from build123d import *

# Parameters (mm, degrees)
F1_DEPTH       = 31.75
F4_D           = 6.985
F4_DEPTH       = 12.7
F4_CSINK_D     = 12.7
F4_CSINK_ANGLE = 82
F4_TIP         = 2.098505712
F5_SIZE2       = 0.381
F5_SIZE        = 6.35
F2_W           = 4.7625
F2_H           = 20.32
F6_DEPTH       = 25.4
F7_SIZE2       = 5.08
F7_SIZE        = 0.381
F8_R           = 1.905
F9_T1_DEPTH    = 23.1775
F9_T3_DEPTH    = 27.94
F9_S7_W        = 1.905
F9_S7_H        = 1.905
F9_T8_DEPTH    = 1.905
F9_S13_W       = 1.905
F9_S13_H       = 1.905
F9_T14_DEPTH   = 1.905
F9_S19_W       = 1.905
F9_S19_H       = 1.905
F9_T20_DEPTH   = 1.905
F9_S25_W       = 1.905
F9_S25_H       = 1.905
F9_T26_DEPTH   = 1.905


# Not quite as in the source:
# - a fillet or chamfer that OpenCascade refuses, or shapes differently, is made with other operations: its cross-section is extruded or revolved along the edge and cut away or added


with BuildPart() as f1:
    # F0 (on Right) → F1 (new body, symmetric)
    with BuildSketch(Plane.YZ):
        Polygon((-12.7, 0), (-12.7, 20.32), (12.7, 20.32), (12.7, 0), (17.4625, 0), (17.4625, 25.0825), (-17.4625, 25.0825), (-17.4625, 0), align=None)
    extrude(amount=F1_DEPTH, both=True)

    # F4
    with Locations(Plane.XY.offset(25.0825)):
        with Locations((0, 0)):
            CounterSinkHole(F4_D / 2, F4_CSINK_D / 2, depth=F4_DEPTH, counter_sink_angle=F4_CSINK_ANGLE)
            with Locations((0, 0, -(F4_DEPTH + F4_TIP / 2))):  # 118° drill point
                Cone(0, F4_D / 2, F4_TIP, mode=Mode.SUBTRACT)

    # F5
    f5_edges = [f1.edges().sort_by_distance(p)[0] for p in [
        (0, -12.7, 0),
    ]]
    f5_side = f1.faces().sort_by_distance((0, -12.7, 10.16))[0]
    chamfer(f5_edges, length=F5_SIZE, length2=F5_SIZE2, reference=f5_side)

    # F2 (on face) → F6 (join)
    with BuildSketch(Plane(origin=(-31.75, 0, 0), x_dir=(0, -1, 0), z_dir=(-1, 0, 0))):
        with Locations((-15.08125, 10.16)):
            Rectangle(F2_W, F2_H)
    extrude(amount=F6_DEPTH)

    # F7
    f7_edges = [f1.edges().sort_by_distance(p)[0] for p in [
        (-12.7, 12.7, 0),
    ]]
    chamfer(f7_edges, length=F7_SIZE, length2=F7_SIZE2)

    # F8
    f8_edges = [f1.edges().sort_by_distance(p)[0] for p in [
        (-31.75, 0, 25.0825),
        (-31.75, 15.08125, 20.32),
        (-57.15, 15.08125, 20.32),
        (31.75, 0, 25.0825),
        (0, 17.4625, 25.0825),
        (-31.75, 17.4625, 22.70125),
        (-44.45, 17.4625, 20.32),
        (0, -17.4625, 25.0825),
    ]]
    fillet(f8_edges, radius=F8_R)

    # F9: fillet of radius 1.905 on 4 edges, made by hand

    # F9_s2 → F9_t1 (cut)
    with BuildSketch(Plane.XY.offset(-4.7625)):
        with BuildLine():
            ThreePointArc((-55.245, 17.4625), (-56.5920384182, 16.9045384182), (-57.15, 15.5575))
            Line((-57.15, 15.5575), (-57.15, 17.4625))
            Line((-57.15, 17.4625), (-55.245, 17.4625))
        make_face()
    extrude(amount=F9_T1_DEPTH, mode=Mode.SUBTRACT)

    # F9_s4 → F9_t3 (cut)
    with BuildSketch(Plane.XY.offset(-4.7625)):
        with BuildLine():
            ThreePointArc((31.75, 15.5575), (31.1920384182, 16.9045384182), (29.845, 17.4625))
            Line((29.845, 17.4625), (31.75, 17.4625))
            Line((31.75, 17.4625), (31.75, 15.5575))
        make_face()
        with BuildLine():
            ThreePointArc((-29.845, -17.4625), (-31.1920384182, -16.9045384182), (-31.75, -15.5575))
            Line((-31.75, -15.5575), (-31.75, -17.4625))
            Line((-31.75, -17.4625), (-29.845, -17.4625))
        make_face()
        with BuildLine():
            ThreePointArc((31.75, -15.5575), (31.1920384182, -16.9045384182), (29.845, -17.4625))
            Line((29.845, -17.4625), (31.75, -17.4625))
            Line((31.75, -17.4625), (31.75, -15.5575))
        make_face()
    extrude(amount=F9_T3_DEPTH, mode=Mode.SUBTRACT)


with BuildPart() as f9_tool6:
    # F9_s7 → F9_t8 (new body)
    with BuildSketch(Plane.YZ.offset(29.845)):
        with Locations((-16.51, 24.13)):
            Rectangle(F9_S7_W, F9_S7_H)
    extrude(amount=F9_T8_DEPTH)

    # F9_s9 → F9_t10 (revolve, cut)
    with BuildSketch(Plane(origin=(29.845, -15.5575, 23.1775), x_dir=(0, 0.7071067812, -0.7071067812), z_dir=(0, -0.7071067812, -0.7071067812))):
        with BuildLine():
            ThreePointArc((0, -1.905), (1.905, 0), (0, 1.905))
            Line((0, 1.905), (0, -1.905))
        make_face()
    revolve(axis=Axis((29.845, -15.5575, 23.1775), (1, 0, 0)), mode=Mode.SUBTRACT)


with BuildPart() as f1_1:
    add(f1.part)

    # F9_t5: cut F9_tool6
    add(f9_tool6.part, mode=Mode.SUBTRACT)


with BuildPart() as f9_tool12:
    # F9_s13 → F9_t14 (new body)
    with BuildSketch(Plane.XZ.offset(15.5575)):
        with Locations((-30.7975, 24.13)):
            Rectangle(F9_S13_W, F9_S13_H)
    extrude(amount=F9_T14_DEPTH)

    # F9_s15 → F9_t16 (revolve, cut)
    with BuildSketch(Plane(origin=(-29.845, -15.5575, 23.1775), x_dir=(0.7071067812, 0, -0.7071067812), z_dir=(-0.7071067812, 0, -0.7071067812))):
        with BuildLine():
            ThreePointArc((0, -1.905), (1.905, 0), (0, 1.905))
            Line((0, 1.905), (0, -1.905))
        make_face()
    revolve(axis=Axis((-29.845, -15.5575, 23.1775), (0, -1, 0)), mode=Mode.SUBTRACT)


with BuildPart() as f1_2:
    add(f1_1.part)

    # F9_t11: cut F9_tool12
    add(f9_tool12.part, mode=Mode.SUBTRACT)


with BuildPart() as f9_tool18:
    # F9_s19 → F9_t20 (new body)
    with BuildSketch(Plane.YZ.offset(29.845)):
        with Locations((16.51, 24.13)):
            Rectangle(F9_S19_W, F9_S19_H)
    extrude(amount=F9_T20_DEPTH)

    # F9_s21 → F9_t22 (revolve, cut)
    with BuildSketch(Plane(origin=(29.845, 15.5575, 23.1775), x_dir=(0, -0.7071067812, -0.7071067812), z_dir=(0, -0.7071067812, 0.7071067812))):
        with BuildLine():
            ThreePointArc((0, -1.905), (1.905, 0), (0, 1.905))
            Line((0, 1.905), (0, -1.905))
        make_face()
    revolve(axis=Axis((29.845, 15.5575, 23.1775), (1, 0, 0)), mode=Mode.SUBTRACT)


with BuildPart() as f1_3:
    add(f1_2.part)

    # F9_t17: cut F9_tool18
    add(f9_tool18.part, mode=Mode.SUBTRACT)


with BuildPart() as f9_tool24:
    # F9_s25 → F9_t26 (new body)
    with BuildSketch(Plane.XZ.offset(-15.5575)):
        with Locations((-56.1975, 19.3675)):
            Rectangle(F9_S25_W, F9_S25_H)
    extrude(amount=-F9_T26_DEPTH)

    # F9_s27 → F9_t28 (revolve, cut)
    with BuildSketch(Plane(origin=(-55.245, 15.5575, 18.415), x_dir=(0.7071067812, 0, -0.7071067812), z_dir=(0.7071067812, 0, 0.7071067812))):
        with BuildLine():
            ThreePointArc((0, -1.905), (1.905, 0), (0, 1.905))
            Line((0, 1.905), (0, -1.905))
        make_face()
    revolve(axis=Axis((-55.245, 15.5575, 18.415), (0, 1, 0)), mode=Mode.SUBTRACT)


with BuildPart() as f1_4:
    add(f1_3.part)

    # F9_t23: cut F9_tool24
    add(f9_tool24.part, mode=Mode.SUBTRACT)

    # F10: F1 across plane


with BuildPart() as f1_5:
    add(f1_4.part)
    add(f1_4.part.mirror(Plane.YZ))


solid = f1_5.part
Verification items for the finished model (mm, model axes). A direction names the side the tool comes from. Round coordinates to 2 decimals unless told otherwise and drop trailing zeros. Write each question's results on one line, items separated by ' | '.
1) Mould release check, pull along Y, two halves, no side actions. Record for faces 1 (the cylindrical face through (-31.177, 16.919, 22.708)), 2 (the cylindrical face through (56.607, 14.109, 19.747)), 3 (the flat face through (0.444, -12.893, 3.131)): released by +Y, released by -Y, zero draft, split by the parting line, or undercut.
Checks:
face 1: released by +Y | face 2: zero draft | face 3: undercut
2) Gauge pin test, flat ends, axial feed: P1, Ø10, axis at y = 6.5, z = 4, coming from the -X side; P2, Ø1.4, axis at x = -47.5, y = 14, coming from the +Z side; P3, Ø5, axis at x = 38.5, z = 15, coming from the -Y side; P4, Ø10, axis at x = 30, y = 4, coming from the -Z side. Record the tip position at first contact, or that the pin passes through.
Checks:
P1: passes through | P2: stops at z = 20.32 | P3: stops at y = 12.7 | P4: stops at z = 20.32
3) Access from +Z, -Z, +X, -X, +Y, -Y to the whole of each face (thin tool, end or side, straight path). Record for faces 4 (the cylindrical face through (-44.601, 16.919, 19.747)), 5 (the flat face through (0, 5, 20.32)), 6 (the flat face through (44, 14, 20.32)), 7 (the cylindrical face through (31.207, 16.89, 22.695)).
Checks:
face 4: +Z, -X, +Y | face 5: -Z, +X, -X | face 6: +Z, +X, +Y, -Y | face 7: +Z, +X, +Y
4) Scan lines: L1, parallel to Y at x = -10.5, z = 13.25; L2, parallel to X at y = 0, z = 20.95; L3, parallel to Y at x = 0, z = 21.5. Record each from-to range of solid material in increasing order. Write a range as from..to.
Checks:
L1: y = -17.46..-12.7, 12.7..17.46 | L2: x = -31.75..-3.49, 3.49..31.75 | L3: y = -17.46..-3.49, 3.49..17.46
